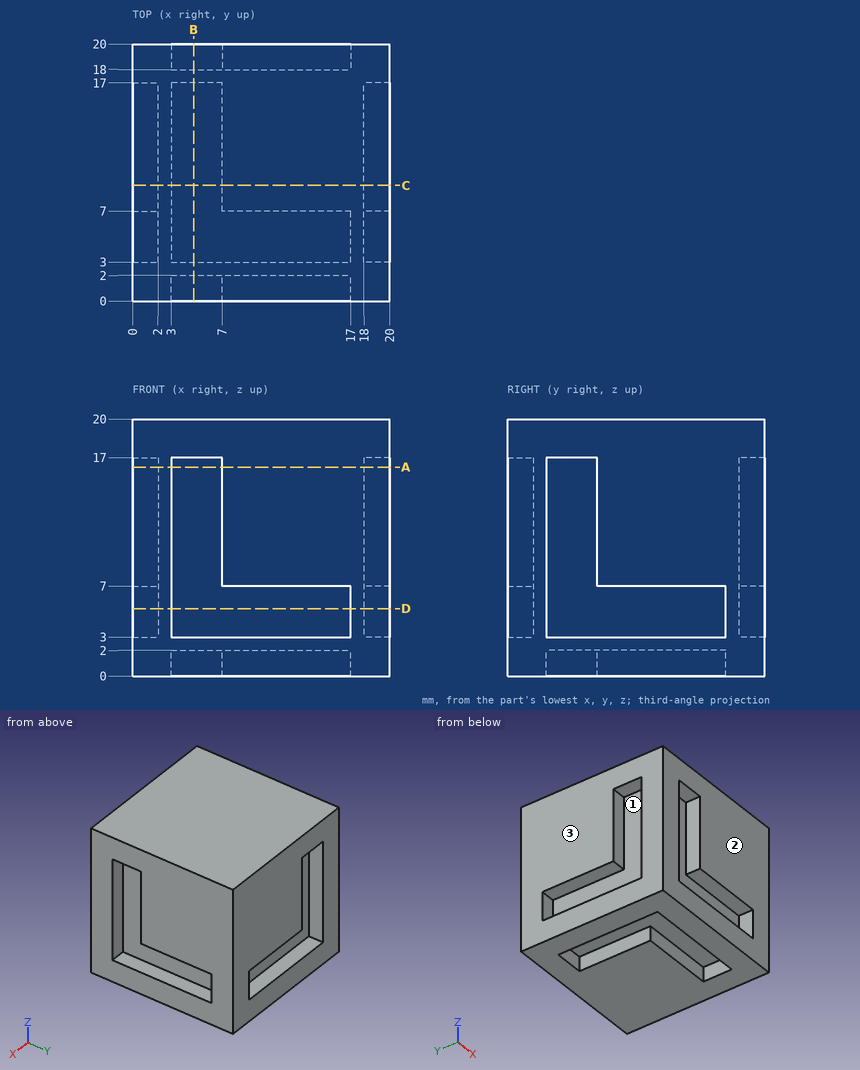
Here's the drawing with two shaded views (mm, measured from the low corner). I have some questions. Round coordinates to 2 decimals unless told otherwise and drop trailing zeros. Write each loop counter-clockwise with the first axis right and the second up, starting at its lowest first coordinate (ties: lowest second). Pieces come first, ordered by that corner, then holes.
(1) Suppose I cut it at C-C on y = 9. Write out the boundary of the cut face in (x, z), and give its area (3 significant figures).
Findings below:
outline: (0, 0) - (3, 0) - (3, 2) - (7, 2) - (7, 0) - (20, 0) - (20, 3) - (18, 3) - (18, 7) - (20, 7) - (20, 20) - (0, 20) - (0, 7) - (2, 7) - (2, 3) - (0, 3) - close
area: 376 mm2
(2) Thinking about a two-plate mould opening in Y: for the marked faces 1, 2 and 3, which applies, +Y half, -Y half, draft (parallel to the pull), parting line (faces both ways), or undercut?
Findings below:
face 1: undercut
face 2: -Y half
face 3: draft
(3) Suppose I cut it at B-B on x = 4.75. Write out the boundary of the cut face in (y, z).
Findings below:
outline: (0, 0) - (3, 0) - (3, 2) - (17, 2) - (17, 0) - (20, 0) - (20, 3) - (18, 3) - (18, 17) - (20, 17) - (20, 20) - (0, 20) - (0, 17) - (2, 17) - (2, 3) - (0, 3) - close
(4) If I drill on probe 1 along Y at (x, z) = (19, 16); probe 2 along Y at (x, z) = (6.75, 3.5), over which ranges is the centre line in solid material (lowest first)?
Findings below:
probe 1: y = 0 to 3, 7 to 20
probe 2: y = 2 to 18
(5) Suppose I cut it at A-A on z = 16.25. Write out the boundary of the cut face in (x, y), and give its area (3 significant figures).
Findings below:
outline: (0, 0) - (3, 0) - (3, 2) - (7, 2) - (7, 0) - (20, 0) - (20, 3) - (18, 3) - (18, 7) - (20, 7) - (20, 20) - (7, 20) - (7, 18) - (3, 18) - (3, 20) - (0, 20) - (0, 7) - (2, 7) - (2, 3) - (0, 3) - close
area: 368 mm2
(6) Suppose I cut it at D-D on z = 5.25. Write out the boundary of the cut face in (x, y).
Findings below:
outline: (0, 0) - (3, 0) - (3, 2) - (17, 2) - (17, 0) - (20, 0) - (20, 3) - (18, 3) - (18, 17) - (20, 17) - (20, 20) - (17, 20) - (17, 18) - (3, 18) - (3, 20) - (0, 20) - (0, 17) - (2, 17) - (2, 3) - (0, 3) - close
